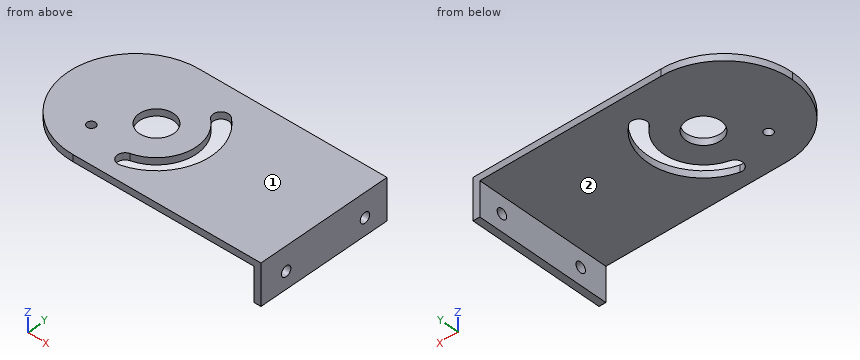
```python
from build123d import *

# Parameters (mm, degrees)
SKETCH_2_W          = 75
SKETCH_2_H          = 40
EXTRUDE_1_DEPTH     = 2
SKETCH_3_R          = 5.05
SKETCH_3_R_2        = 1.25
CUT_EXTRUDE_1_DEPTH = 86.023526156
FILLET_1_R          = 20
SKETCH_7_W          = 2
SKETCH_7_H          = 40
EXTRUDE_3_DEPTH     = 10
SKETCH_10_R         = 1.5
CUT_EXTRUDE_4_DEPTH = 84.839131675


with BuildPart() as part:
    # 草图2 → 凸台-拉伸1 (new body)
    with BuildSketch(Plane.XY):
        with Locations((37.5, 20)):
            Rectangle(SKETCH_2_W, SKETCH_2_H)
    extrude(amount=EXTRUDE_1_DEPTH)

    # 草图3 → 切除-拉伸1 (cut, through all)
    with BuildSketch(Plane(origin=(0, 0, 0), x_dir=(-1, 0, 0), z_dir=(0, 0, -1))):
        with Locations((-26, 20)):
            Circle(SKETCH_3_R)
        with Locations((-16, 10.202041029)):
            Circle(SKETCH_3_R_2)
        with BuildLine():
            ThreePointArc((-36.446428571, 32.447274003), (-41.830655455, 16.332187591), (-29.908043377, 4.226931276))
            ThreePointArc((-29.908043377, 4.226931276), (-27.182966317, 5.86978094), (-28.82581598, 8.594858))
            ThreePointArc((-28.82581598, 8.594858), (-37.446781637, 17.347889489), (-33.553571429, 29.000336587))
            ThreePointArc((-33.553571429, 29.000336587), (-33.276531292, 32.170233866), (-36.446428571, 32.447274003))
        make_face()
    extrude(amount=-CUT_EXTRUDE_1_DEPTH, mode=Mode.SUBTRACT)

    # 圆角1
    fillet_1_edges = [part.edges().sort_by_distance(p)[0] for p in [
        (0, 40, 1),
        (0, 0, 1),
    ]]
    fillet(fillet_1_edges, radius=FILLET_1_R - 0.0001)  # a hair under: the kernel refuses the full size

    # 草图7 → 凸台-拉伸3 (add)
    with BuildSketch(Plane(origin=(0, 0, 0), x_dir=(-1, 0, 0), z_dir=(0, 0, -1))):
        with Locations((-74, 20)):
            Rectangle(SKETCH_7_W, SKETCH_7_H)
    extrude(amount=EXTRUDE_3_DEPTH)

    # 草图10 → 切除-拉伸4 (cut, through all)
    with BuildSketch(Plane.ZY.offset(-73)):
        with Locations((-5, 33)):
            Circle(SKETCH_10_R)
        with Locations((-5, 8)):
            Circle(SKETCH_10_R)
    extrude(amount=-CUT_EXTRUDE_4_DEPTH, mode=Mode.SUBTRACT)


solid = part.part
```
The model under review builds one solid part; all positions refer to its coordinate system, in mm. Face numbers are marked on the shaded views. A direction names the side the tool comes from. Give positions to 0.01 mm unless a question says otherwise; leave off trailing zeros. Loops run counter-clockwise (first coordinate to the right, second up) from the corner with the lowest first, then second, coordinate; pieces in that order, holes last. Notation, with made-up numbers: (59, -35.75) - (102, -35.75) arc R29 cw to (102, 3.25) - close; hole circle Ø8 at (43, 2.25). An arc over 180 degrees is marked (long way). Answer as a JSON object with one key per item and string values.
Q1. For the marked faces 1 and 2, list the 3-axis set-ups (+Z, -Z, +X, -X, +Y, -Y) from which the entire face can be reached by the end or side of a thin tool; tool diameter is ignored.
Worked out:
{"face 1": "+Z, +X, -X, +Y, -Y", "face 2": "-Z, -X, +Y, -Y"}
Q2. Add section B-B on x = 26. State the section outline as (y, z) points, plus the area to 3 significant figures.
Worked out:
{"outline": "(0, 0) - (14.95, 0) - (14.95, 2) - (0, 2) - close; (25.05, 0) - (40, 0) - (40, 2) - (25.05, 2) - close", "area": "59.8 mm^2"}
Q3. To check wall thickness, follow line 1 along Y through (x, z) = (73.75, -5); line 2 along Y through (x, z) = (26, 0.6); line 3 along X through (y, z) = (23.5, 1). State the ranges of each line that lie inside material, in increasing order.
Worked out:
{"line 1": "y = 0 to 6.5, 9.5 to 31.5, 34.5 to 40", "line 2": "y = 0 to 14.95, 25.05 to 40", "line 3": "x = 0.31 to 22.36, 29.64 to 37.22, 41.87 to 75"}
Q4. Add section A-A on z = -5. State the section outline as (x, y) points, plus the area to 3 significant figures.
Worked out:
{"outline": "(73, 0) - (75, 0) - (75, 6.5) - (73, 6.5) - close; (73, 9.5) - (75, 9.5) - (75, 31.5) - (73, 31.5) - close; (73, 34.5) - (75, 34.5) - (75, 40) - (73, 40) - close", "area": "68.0 mm^2"}
Q5. Add section C-C on y = 13.5. State the section outline as (x, z) points, plus the area to 3 significant figures.
Worked out:
{"outline": "(1.09, 0) - (35.79, 0) - (35.79, 2) - (1.09, 2) - close; (40.89, 0) - (73, 0) - (73, -10) - (75, -10) - (75, 2) - (40.89, 2) - close", "area": "158 mm^2"}
Q6. Add section D-D on z = 0.75. Count the separate pieces of the cut face and the enclosed holes in it, plus the area to 3 significant figures.
Worked out:
{"separate pieces": "1", "enclosed holes": "3", "area": "2,590 mm^2"}
Q7. Insertion check: pin 1 (5 mm diameter, centred on y = 29, z = -6.5, fed in from -X); pin 2 (9 mm diameter, centred on x = 26, y = 20, fed in from +Z); pin 3 (3 mm diameter, centred on x = 16, y = 10.2, fed in from -Z). Each pin has a flat end and moves straight along its axis. Give the tip position at first contact, or say it passes through.
Worked out:
{"pin 1": "stops at x = 73", "pin 2": "passes through", "pin 3": "stops at z = 0"}
